Read the model definition and answer for the solid it produces. Units are mm, in the model's axes. Face numbers are marked on the shaded views. Coordinates: 2 decimals unless noted, no trailing zeros. Order: outer loops, then holes, each group sorted by start corner. A loop starts at its lowest first (then second) coordinate and runs counter-clockwise, first axis right, second up.
```python
from build123d import *

# Parameters (mm, degrees)
F0_R     = 5
F0_R_2   = 3.5
F1_DEPTH = 4
F2_R     = 5


with BuildPart() as f1:
    # F0 (on Top) → F1 (new body)
    with BuildSketch(Plane.XY):
        with BuildLine():
            ThreePointArc((-80, -102), (-79.12132, -104.12132), (-77, -105))
            Line((-77, -105), (-33, -105))
            ThreePointArc((-33, -105), (-30.87868, -104.12132), (-30, -102))
            Line((-30, -102), (-30, -53))
            ThreePointArc((-30, -53), (-29.12132, -50.87868), (-27, -50))
            Line((-27, -50), (27, -50))
            ThreePointArc((27, -50), (29.12132, -50.87868), (30, -53))
            Line((30, -53), (30, -102))
            ThreePointArc((30, -102), (30.87868, -104.12132), (33, -105))
            Line((33, -105), (77, -105))
            ThreePointArc((77, -105), (79.12132, -104.12132), (80, -102))
            Line((80, -102), (80, -20))
            Line((80, -20), (45, -20))
            Line((45, -20), (45, 20))
            Line((45, 20), (80, 20))
            Line((80, 20), (80, 102))
            ThreePointArc((80, 102), (79.12132, 104.12132), (77, 105))
            Line((77, 105), (33, 105))
            ThreePointArc((33, 105), (30.87868, 104.12132), (30, 102))
            Line((30, 102), (30, 53))
            ThreePointArc((30, 53), (29.12132, 50.87868), (27, 50))
            Line((27, 50), (-27, 50))
            ThreePointArc((-27, 50), (-29.12132, 50.87868), (-30, 53))
            Line((-30, 53), (-30, 102))
            ThreePointArc((-30, 102), (-30.87868, 104.12132), (-33, 105))
            Line((-33, 105), (-77, 105))
            ThreePointArc((-77, 105), (-79.12132, 104.12132), (-80, 102))
            Line((-80, 102), (-80, -102))
        make_face()
        with BuildLine():
            Line((-69.994725, -89.77039), (-69.994725, -75.22961))
            ThreePointArc((-69.994725, -75.22961), (-70, -75), (-69.994725, -74.77039))
            ThreePointArc((-69.994725, -74.77039), (-65, -70), (-60.005275, -74.77039))
            Line((-60.005275, -74.77039), (-60.005275, -89.77039))
            ThreePointArc((-60.005275, -89.77039), (-64.77039, -94.994725), (-69.994725, -90.22961))
            ThreePointArc((-69.994725, -90.22961), (-70, -90), (-69.994725, -89.77039))
        make_face(mode=Mode.SUBTRACT)
        with Locations((-65, -45)):
            Circle(F0_R, mode=Mode.SUBTRACT)
        with Locations((-36.5, -36.5)):
            Circle(F0_R_2, mode=Mode.SUBTRACT)
        with BuildLine():
            ThreePointArc((69.994725, -74.77039), (70, -75), (69.994725, -75.22961))
            Line((69.994725, -75.22961), (69.994725, -89.77039))
            ThreePointArc((69.994725, -89.77039), (70, -90), (69.994725, -90.22961))
            ThreePointArc((69.994725, -90.22961), (64.77039, -94.994725), (60.005275, -89.77039))
            Line((60.005275, -89.77039), (60.005275, -74.77039))
            ThreePointArc((60.005275, -74.77039), (65, -70), (69.994725, -74.77039))
        make_face(mode=Mode.SUBTRACT)
        with Locations((36.5, -36.5)):
            Circle(F0_R_2, mode=Mode.SUBTRACT)
        with Locations((65, -45)):
            Circle(F0_R, mode=Mode.SUBTRACT)
        with Locations((-65, 45)):
            Circle(F0_R, mode=Mode.SUBTRACT)
        with Locations((-36.5, 36.5)):
            Circle(F0_R_2, mode=Mode.SUBTRACT)
        with BuildLine():
            ThreePointArc((-69.994725, 90.22961), (-64.77039, 94.994725), (-60.005275, 89.77039))
            Line((-60.005275, 89.77039), (-60.005275, 74.77039))
            ThreePointArc((-60.005275, 74.77039), (-65, 70), (-69.994725, 74.77039))
            ThreePointArc((-69.994725, 74.77039), (-70, 75), (-69.994725, 75.22961))
            Line((-69.994725, 75.22961), (-69.994725, 89.77039))
            ThreePointArc((-69.994725, 89.77039), (-70, 90), (-69.994725, 90.22961))
        make_face(mode=Mode.SUBTRACT)
        with Locations((36.5, 36.5)):
            Circle(F0_R_2, mode=Mode.SUBTRACT)
        with Locations((65, 45)):
            Circle(F0_R, mode=Mode.SUBTRACT)
        with BuildLine():
            Line((69.994725, 89.77039), (69.994725, 75.22961))
            ThreePointArc((69.994725, 75.22961), (70, 75), (69.994725, 74.77039))
            ThreePointArc((69.994725, 74.77039), (65, 70), (60.005275, 74.77039))
            Line((60.005275, 74.77039), (60.005275, 89.77039))
            ThreePointArc((60.005275, 89.77039), (64.77039, 94.994725), (69.994725, 90.22961))
            ThreePointArc((69.994725, 90.22961), (70, 90), (69.994725, 89.77039))
        make_face(mode=Mode.SUBTRACT)
    extrude(amount=F1_DEPTH)

    # F2
    f2_edges = [f1.edges().sort_by_distance(p)[0] for p in [
        (80, -20, 2),
        (45, -20, 2),
        (45, 20, 2),
        (80, 20, 2),
    ]]
    fillet(f2_edges, radius=F2_R)


solid = f1.part
```
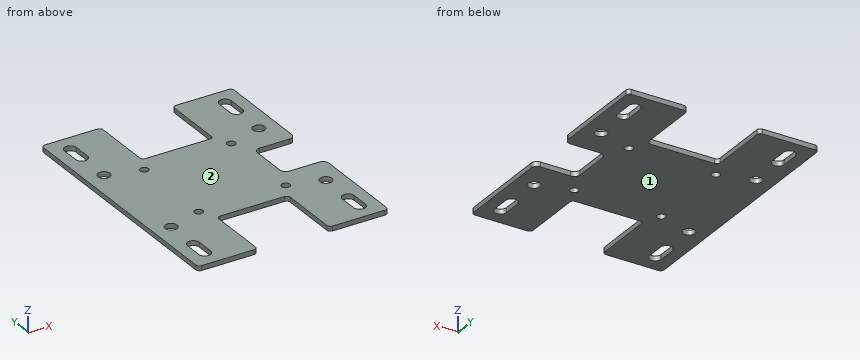
1) Determine the mould class of the marked faces 1 and 2 for opening direction Z: pulls with the +Z half, pulls with the -Z half, needs draft (parallel to the pull), parting line crosses it, or undercut.
A:
face 1: pulls with the -Z half
face 2: pulls with the +Z half
2) Straight lines are drawn through the part: line 1 (Y direction, x = -36.5, z = 1.4); line 2 (X direction, y = -46.5, z = 0.7); line 3 (Y direction, x = 66, z = 3.05). For each, find the intervals that lie inside material, in ascending order.
A:
line 1: y = -105 to -40, -33 to 33, 40 to 105
line 2: x = -80 to -69.77, -60.23 to 60.23, 69.77 to 80
line 3: y = -105 to -94.9, -70.1 to -49.9, -40.1 to -20, 20 to 40.1, 49.9 to 70.1, 94.9 to 105
3) A cutting plane is placed at B-B, the plane y = -66. Determine the outline of the cut face in (x, z).
A:
outline: (-80, 0) - (-30, 0) - (-30, 4) - (-80, 4) - close; (30, 0) - (80, 0) - (80, 4) - (30, 4) - close
4) A flat-ended cylindrical pin translates along its axis: pin 1 Ø1.2 at (x, z) = (9.5, 2.5) entering from +Y. Find the tip coordinate at first contact, or state that the pin passes through.
A:
pin 1: stops at y = 50
5) A cutting plane is placed at C-C, the plane y = 45. Determine the outline of the cut face in (x, z).
A:
outline: (-80, 0) - (-70, 0) - (-70, 4) - (-80, 4) - close; (-60, 0) - (60, 0) - (60, 4) - (-60, 4) - close; (70, 0) - (80, 0) - (80, 4) - (70, 4) - close
6) A cutting plane is placed at A-A, the plane x = 65. Determine the outline of the cut face in (y, z).
A:
outline: (-105, 0) - (-95, 0) - (-95, 4) - (-105, 4) - close; (-70, 0) - (-50, 0) - (-50, 4) - (-70, 4) - close; (-40, 0) - (-20, 0) - (-20, 4) - (-40, 4) - close; (20, 0) - (40, 0) - (40, 4) - (20, 4) - close; (50, 0) - (70, 0) - (70, 4) - (50, 4) - close; (95, 0) - (105, 0) - (105, 4) - (95, 4) - close
7) A cutting plane is placed at D-D, the plane x = 36.5. Determine the outline of the cut face in (y, z).
A:
outline: (-105, 0) - (-40, 0) - (-40, 4) - (-105, 4) - close; (-33, 0) - (33, 0) - (33, 4) - (-33, 4) - close; (40, 0) - (105, 0) - (105, 4) - (40, 4) - close
